Check sheet for the modelled part. Datum: model origin and axes. Units: mm. A direction names the side the tool comes from. Give positions to 0.01 mm unless a question says otherwise; leave off trailing zeros. Write each loop counter-clockwise with the first axis right and the second up, starting at its lowest first coordinate (ties: lowest second). Pieces come first, ordered by that corner, then holes. Notation, with made-up numbers: (4, 73.25) -> (20, 73.25) arc R20 cw to (20, 108.25) -> close; hole circle Ø4 at (21, 51.25). An arc over 180 degrees is marked (long way). Write each question's results on one line, items separated by ' | '. Start each with the question number.
```python
from build123d import *

# Parameters (mm, degrees)
F1_DEPTH = 15


# Not quite as in the source:
# - ends of sketch curves that miss each other by under 0.0002 mm in the source are joined


with BuildPart() as f1:
    # F0 (on Right) → F1 (new body)
    with BuildSketch(Plane.YZ):
        Polygon((57.2133171244, 7), (96.8499479096, 0), (96.8499479096, 22), (88.8499479096, 22), (88.8499479096, 7), align=None)
        Polygon((-129.6450851485, 0), (96.8499479096, 0), (57.2133171244, 7), (-93.3098772168, 7), (-103.3098761737, 7), (-113.3098740876, 7), (-123.3098730445, 7), (-129.6450851485, 7), align=None)
        Polygon((-129.6450851485, 40), (57.2133171244, 7), (88.8499479096, 7), (-137.6450851485, 47), (-137.6450851485, 0), (-129.6450851485, 0), (-129.6450851485, 7), align=None)
        Polygon((-123.3098730445, 14), (-123.3098730445, 7), (-113.3098740876, 7), (-113.3098730445, 14), (-116.3098730445, 14), (-116.3098730445, 12), (-114.8098730445, 12), (-114.8098730445, 9), (-121.8098730445, 9), (-121.8098730445, 12), (-120.3098730445, 12), (-120.3098730445, 14), align=None)
        Polygon((-113.3098740876, 7), (-103.3098761737, 7), (-103.3098751307, 14), (-106.3098751307, 14), (-106.3098751307, 12), (-104.8098751307, 12), (-104.8098751307, 9), (-111.8098751307, 9), (-111.8098751307, 12), (-110.3098751307, 12), (-110.3098751307, 14), (-113.3098751307, 14), align=None)
        Polygon((-103.3098761737, 7), (-93.3098772168, 7), (-93.3098772168, 14), (-96.3098772168, 14), (-96.3098772168, 12), (-94.8098772168, 12), (-94.8098772168, 9), (-101.8098772168, 9), (-101.8098772168, 12), (-100.3098772168, 12), (-100.3098772168, 14), (-103.3098772168, 14), align=None)
    extrude(amount=F1_DEPTH)


solid = f1.part
```
Item 1: Section check A-A on z = 36. Record the boundary of the cut face in (x, y), then the cut area to 3 significant figures.
Item 2: Thickness scan on probe 1 along Z at (x, y) = (4.5, -101.5); probe 2 along Z at (x, y) = (10.5, 0); probe 3 along Z at (x, y) = (11, 54). Record the ranges inside material, lowest first. Write a range as from..to.
Item 3: Section check B-B on y = 4. Record the boundary of the cut face in (x, z).
Item 4: Depth check by flat-ended pin: pin 1 Ø4 at (x, y) = (5.5, -88) entering from +Z; pin 2 Ø0.9 at (x, y) = (10, -122.5) entering from +Z; pin 3 Ø7.5 at (x, y) = (4.5, -99.5) entering from +Z. Enter the tip coordinate at first touch or a pass-through.
Item 5: Mould release check, pull along Y, two halves, no side actions. Record for faces 1 (the flat face through (7, 93, 22)), 2 (the flat face through (7, -108, 9)), 3 (the flat face through (7, 96.85, 11)), 4 (the flat face through (7, -103, 14)): pulls with the +Y half, pulls with the -Y half, needs draft (parallel to the pull), parting line crosses it, or undercut.
Item 6: Set-up check for faces 5 (the flat face through (7, 88.85, 15)), 6 (the flat face through (7, -22, 0)), 7 (the flat face through (7, -17, 7)): record each of +Z, -Z, +X, -X, +Y, -Y from which the full face is reachable in a straight line by a thin tool's end or side.
Item 7: Section check C-C on z = 17.5. Record the boundary of the cut face in (x, y) (3 decimals).
Item 8: Section check D-D on y = 77.5. Record the boundary of the cut face in (x, z).
Check sheet entries:
1) outline: (0, -137.65) -> (15, -137.65) -> (15, -129.65) -> (0, -129.65) -> close; (0, -107) -> (15, -107) -> (15, -75.36) -> (0, -75.36) -> close | area: 595 mm^2
2) probe 1: z = 0..9, 12..14, 35.03..40.62 | probe 2: z = 0..7, 17.1..22.69 | probe 3: z = 0..7, 7.57..13.15
3) outline: (0, 0) -> (15, 0) -> (15, 7) -> (0, 7) -> close; (0, 16.4) -> (15, 16.4) -> (15, 21.98) -> (0, 21.98) -> close
4) pin 1: stops at z = 38.59 | pin 2: stops at z = 44.4 | pin 3: stops at z = 40.93
5) face 1: needs draft | face 2: undercut | face 3: pulls with the +Y half | face 4: undercut
6) face 5: +Z, +X, -X | face 6: -Z, +X, -X, +Y, -Y | face 7: +X, -X
7) outline: (0, -137.645) -> (15, -137.645) -> (15, -129.645) -> (0, -129.645) -> close; (0, -2.242) -> (15, -2.242) -> (15, 29.395) -> (0, 29.395) -> close; (0, 88.85) -> (15, 88.85) -> (15, 96.85) -> (0, 96.85) -> close
8) outline: (0, 0) -> (15, 0) -> (15, 9) -> (0, 9) -> close
